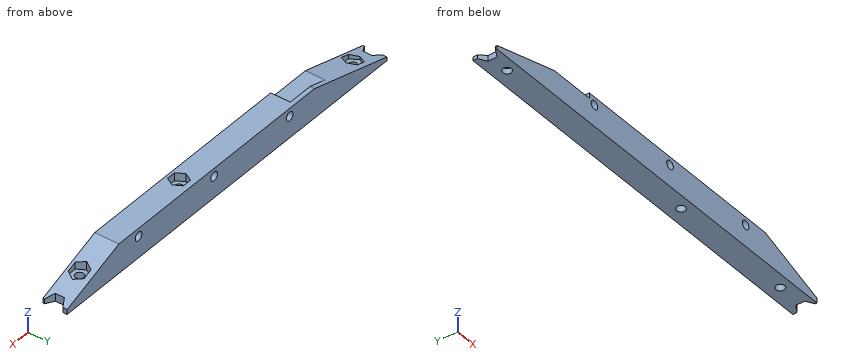
Autodesk Inventor part; units mm, degrees
ref_plane "YZ Plane" through (0, 0, 0) normal (1, 0, 0) x (0, 1, 0)
ref_plane "XZ Plane" through (0, 0, 0) normal (0, 1, 0) x (-1, 0, 0)
ref_plane "XY Plane" through (0, 0, 0) normal (0, 0, 1) x (1, 0, 0)
sketch "Sketch1" plane through (0, 0, 0) normal (0, 0, 1) x (1, 0, 0)
  line L0 (0, 0) -> (164.5, 0)
  line L1 (164.5, 0) -> (164.5, 9)
  line L2 (164.5, 9) -> (0, 9)
  line L3 (0, 9) -> (0, 0)
  circle A0 centre (99, 4) radius 1.6
  circle A1 centre (159.5, 4) radius 1.6
  circle A2 centre (147, 4) radius 1.6
  circle A3 centre (15, 4) radius 1.6
  circle A4 centre (5, 4) radius 1.6
  dimension "d1" = 9
  dimension "d2" = 90
  dimension "d6" = 3.2
  dimension "d7" = 3.2
  dimension "d9" = 60.5
  dimension "d26" = 3.2
  dimension "d27" = 48
  dimension "d28" = 3.2
  dimension "d32" = 15
  dimension "d33" = 5
  dimension "d61" = 3.2
  dimension "d62" = 10
  dimension "d63" = 12.5
  dimension "d108" = 4
  dimension "d109" = 4
  dimension "d111" = 4
  dimension "d112" = 4
  dimension "d113" = 4
ref_plane "Work Plane2" through (0, 0, 0) normal (0, -1, 0) x (1, 0, 0)
sketch "Sketch2" plane through (0, 0, 0) normal (0, -1, 0) x (1, 0, 0)
  circle A0 centre (52, 8) radius 1.6
  circle A1 centre (125, 8) radius 1.6
  circle A2 centre (88.5, 8) radius 1.6
  point P0 (0, 0)
  point P1 (52, 0)
  dimension "d13" = 3.2
  dimension "d15" = 3.2
  dimension "d17" = 3.2
  dimension "d18" = 36.5
  dimension "d64" = 52
  dimension "d65" = 36.5
  dimension "d114" = 8
  dimension "d115" = 73
ref_plane "Work Plane1" through (0, 0, 11) normal (0, 0, 1) x (1, 0, 0)
extrude "klocek" add sketch "Sketch1" along normal blind 11
ref_plane "Work Plane3" through (0, 0, 0) normal (0, -1, 0) x (1, 0, 0)
extrude "prowadzenie osi" cut sketch "Sketch2" against normal up to next
ref_plane "Work Plane4" through (0, 0, 0) normal (0, -1, 0) x (1, 0, 0)
sketch "Sketch7" plane through (0, 0, 0) normal (0, -1, 0) x (1, 0, 0)
  line L0 (0, 11) -> (0, 0)
  line L1 (0, 11) -> (164.5, 11)
  line L2 (0, 11) -> (40, 11)
  line L3 (40, 11) -> (0, 0)
  point P0 (0, -1.8333)
  dimension "d86" = 11
  dimension "d87" = 40
sketch "Sketch8" plane through (0, 0, 0) normal (0, -1, 0) x (1, 0, 0)
  line L0 (164.5, 0) -> (164.5, 11)
  line L1 (164.5, 11) -> (164.5, 0)
  line L2 (164.5, 11) -> (0, 11)
  line L3 (164.5, 11) -> (134.5, 11)
  line L4 (134.5, 11) -> (164.5, 0)
  point P0 (0, 0)
  point P1 (40.8333, 11)
  dimension "d80" = 11
  dimension "d81" = 30
extrude "przedni skos" cut sketch "Sketch7" against normal up to next
extrude "tylni skos" cut sketch "Sketch8" against normal up to next
ref_plane "Work Plane7" through (0, 0, 11) normal (0, 0, 1) x (1, 0, 0)
sketch "Sketch5" plane through (0, 0, 11) normal (0, 0, 1) x (1, 0, 0)
  circle A0 centre (99, 4) radius 1.6
  line L0 (95.5936, 4) -> (97.2968, 6.95)
  line L1 (97.2968, 6.95) -> (100.7032, 6.95)
  line L2 (100.7032, 6.95) -> (102.4064, 4)
  line L3 (102.4064, 4) -> (100.7032, 1.05)
  line L4 (100.7032, 1.05) -> (97.2968, 1.05)
  line L5 (97.2968, 1.05) -> (95.5936, 4)
  point P0 (119.5, 5)
  dimension "d98" = 5.9
extrude "hex insert middle" cut sketch "Sketch5" against normal blind 3
ref_plane "Work Plane6" through (0, 0, 11) normal (0, 0, 1) x (1, 0, 0)
sketch "Sketch9" plane through (0, 0, 11) normal (0, 0, 1) x (1, 0, 0)
  circle A0 centre (147, 4) radius 1.6
  line L0 (150.4064, 4) -> (148.7032, 1.05)
  line L1 (148.7032, 1.05) -> (145.2968, 1.05)
  line L2 (145.2968, 1.05) -> (143.5936, 4)
  line L3 (143.5936, 4) -> (145.2968, 6.95)
  line L4 (145.2968, 6.95) -> (148.7032, 6.95)
  line L5 (148.7032, 6.95) -> (150.4064, 4)
  point P0 (0, 0)
  point P1 (153, 5)
  dimension "d99" = 5.9
extrude "hex insert rear 1" cut sketch "Sketch9" against normal blind 6.5
ref_plane "Work Plane5" through (0, 0, 11) normal (0, 0, 1) x (1, 0, 0)
sketch "Sketch10" plane through (0, 0, 11) normal (0, 0, 1) x (1, 0, 0)
  circle A0 centre (159.5, 4) radius 1.6
  line L0 (162.45, 5.7032) -> (162.45, 2.2968)
  line L1 (162.45, 2.2968) -> (159.5, 0.5936)
  line L2 (159.5, 0.5936) -> (156.55, 2.2968)
  line L3 (156.55, 2.2968) -> (156.55, 5.7032)
  line L4 (156.55, 5.7032) -> (159.5, 7.4064)
  line L5 (159.5, 7.4064) -> (162.45, 5.7032)
  line L6 (164.5, 0) -> (134.5, 0)
  point P0 (0, 0)
  dimension "d118" = 5.9
extrude "hex insert rear 2" cut sketch "Sketch10" against normal up to next contours A0 | L0 L1 L2 L3 L4 L5
sketch "Sketch13" plane through (0, 0, 11) normal (0, 0, 1) x (1, 0, 0)
  line L0 (9.54, 0) -> (-1.59, 0)
  line L1 (7.95, 2.2968) -> (5, 0.5936)
  line L2 (5, 0.5936) -> (2.05, 2.2968)
  line L3 (2.05, 2.2968) -> (2.05, 5.7032)
  line L4 (2.05, 5.7032) -> (5, 7.4064)
  line L5 (5, 7.4064) -> (7.95, 5.7032)
  line L6 (7.95, 5.7032) -> (7.95, 2.2968)
  point P0 (0, 0)
  point P1 (5, 4)
  point P2 (5, 4)
  dimension "d117" = 5.9
extrude "hex insert front 1" cut sketch "Sketch13" against normal through all
sketch "Sketch16" plane through (0, 0, 11) normal (0, 0, 1) x (1, 0, 0)
  circle A0 centre (15, 4) radius 1.6
  line L0 (18.4064, 4) -> (16.7032, 1.05)
  line L1 (16.7032, 1.05) -> (13.2968, 1.05)
  line L2 (13.2968, 1.05) -> (11.5936, 4)
  line L3 (11.5936, 4) -> (13.2968, 6.95)
  line L4 (13.2968, 6.95) -> (16.7032, 6.95)
  line L5 (16.7032, 6.95) -> (18.4064, 4)
  point P0 (0, 0)
  dimension "d93" = 5.9
extrude "hex insert front 2" cut sketch "Sketch16" against normal blind 9
sketch "Sketch17" plane through (0, 0, 0) normal (0, 0, -1) x (-1, 0, 0)
  line L0 (0, 9) -> (0, 0)
  line L1 (0, 0) -> (-5, 0)
  line L2 (-5, 0) -> (-5, 10.0042)
  line L3 (-5, 10.0042) -> (0, 10.0042)
  line L4 (0, 10.0042) -> (0, 0)
  point P0 (-5, 7.4064)
extrude "ciecie przod" cut sketch "Sketch17" against normal up to next
sketch "Sketch18" plane through (40, 0, 11) normal (0, -1, 0) x (1, 0, 0)
  line L0 (9.5, 0) -> (9.5, -2)
  line L1 (9.5, -2) -> (-7.5, -2)
  line L2 (-7.5, -2) -> (-7.5, 0)
  line L3 (-7.5, 0) -> (9.5, 0)
  line L4 (94.5, 0) -> (0, 0)
  circle A0 centre (12, -3) radius 1.6
  line L5 (-35, -11) -> (124.5, -11)
  point P0 (-40, -11)
  dimension "d102" = 2
  dimension "d103" = 17
  dimension "d104" = 2.5
extrude "sensor linii" cut sketch "Sketch18" against normal blind 7.3 contours L0 L1 L2 L3
sketch "Sketch21" plane through (0, 0, 0) normal (0, 0, -1) x (-1, 0, 0)
  line L0 (-159.5, 8.9293) -> (-159.5, 0)
  line L1 (-164.5, 0) -> (-134.5, 0)
  line L2 (-159.5, 0) -> (-164.5, 0)
  line L3 (-164.5, 0) -> (-164.5, 9)
  line L4 (-164.5, 9) -> (-159.5, 9)
  line L5 (-159.5, 9) -> (-159.5, 8.9293)
  line L6 (-134.5, 9) -> (-164.5, 9)
  line L7 (-164.5, 9) -> (-164.5, 0)
  point P0 (0, 0)
extrude "ciecie tyl" cut sketch "Sketch21" against normal up to next
properties part number "wheel_support_v4_narrow_with_line_sensor"
The listing builds one solid part. Answer for the finished solid, in the listing's coordinates (mm). Round coordinates to 2 decimals unless told otherwise and drop trailing zeros. Order: outer loops, then holes, each group sorted by start corner. A loop starts at its lowest first (then second) coordinate and runs counter-clockwise, first axis right, second up. Notation, with made-up numbers: (6.5, -1.5) -> (53.5, -1.5) arc R12 cw to (53.5, 4.5) -> close; hole circle Ø4 at (-12, 29.5). An arc over 180 degrees is marked (long way). Answer as CSV lines item,"result". Start each with the question number.
(1) Flat-ended cylindrical pins translate along their axes: pin 1 Ø1.6 at (y, z) = (5, 10) entering from -X; pin 2 Ø3 at (x, y) = (146.5, 4.5) entering from +Z; pin 3 Ø1.6 at (x, z) = (42, 10) entering from -Y. Find the tip coordinate at first contact, or state that the pin passes through.
(2) The part is cut by section A-A (x = 99). Determine the outline of the cut face in (y, z).
(3) Find the intervals of material crossed by probe 1 along Y at (x, z) = (99, 6.5); probe 2 along Z at (x, y) = (125, 5.5); probe 3 along Z at (x, y) = (148.5, 2.25), in increasing order. Write a range as from..to.
(4) The part is cut by section B-B (x = 125). Determine the outline of the cut face in (y, z).
(5) The part is cut by section C-C (x = 147). Determine the outline of the cut face in (y, z).
Evaluation:
1,pin 1,"x = 49.5"
1,pin 2,"z = 4.5"
1,pin 3,"y = 7.3"
2,outline,"(0, 0) -> (2.4, 0) -> (2.4, 8) -> (1.05, 8) -> (1.05, 11) -> (0, 11) -> close; (5.6, 0) -> (9, 0) -> (9, 11) -> (6.95, 11) -> (6.95, 8) -> (5.6, 8) -> close"
3,probe 1,"0..2.4, 5.6..9"
3,probe 2,"0..6.4, 9.6..11"
3,probe 3,"0..4.5"
4,outline,"(0, 0) -> (9, 0) -> (9, 6.4) -> (0, 6.4) -> close; (0, 9.6) -> (9, 9.6) -> (9, 11) -> (0, 11) -> close"
5,outline,"(0, 0) -> (2.4, 0) -> (2.4, 4.5) -> (1.05, 4.5) -> (1.05, 6.42) -> (0, 6.42) -> close; (5.6, 0) -> (9, 0) -> (9, 6.42) -> (6.95, 6.42) -> (6.95, 4.5) -> (5.6, 4.5) -> close"
